Here's how the part is built. I have some questions about the finished solid (model axes, mm). A direction names the side the tool comes from. Round coordinates to 2 decimals unless told otherwise and drop trailing zeros. Write each loop counter-clockwise with the first axis right and the second up, starting at its lowest first coordinate (ties: lowest second). Pieces come first, ordered by that corner, then holes. Notation, with made-up numbers: (66.25, -6.75) - (81.25, -6.75) arc R24 cw to (81.25, 3.25) - close; hole circle Ø7 at (34, 40). An arc over 180 degrees is marked (long way). Write item = value, one per line. Start each with the question number.
Item 1: If I drill on line 1 along Y through (x, z) = (34.5, -9.25); line 2 along X through (y, z) = (-13, 1.25); line 3 along Z through (x, y) = (49, 34), over which ranges is the centre line in solid material (lowest first)? Write a range as [from, to].
Item 2: If we section it at C-C (z = -1.75): Please give me the cut outline in (x, y), and give its area (3 significant figures).
Item 3: If we section it at B-B (x = 4): Please give me the cut outline in (y, z), and give its area (3 significant figures).
Item 4: If we section it at D-D (y = -31): Please give me the cut outline in (x, z), and give its area (3 significant figures).
Item 5: Thinking about a two-plate mould opening in X: for faces 4 (the face through (33, 32.5, -13)), 5 (the face through (48, 20, -13)), 6 (the face through (18, -41, 1)), which applies, pulls with the +X half, pulls with the -X half, needs draft (parallel to the pull), parting line crosses it, or undercut?
Item 6: Which directions (+Z, -Z, +X, -X, +Y, -Y) give clear straight access to the entire face, cutting with the end or side of a thin tool? Please do faces 1 (the face through (0, -37.48, 2)), 2 (the face through (-18, -41, 1)), 3 (the face through (33, -34.5, -13)).
Item 7: If we section it at A-A (y = 11.5): Please give me the cut outline in (x, z), and give its area (3 significant figures).
Item 8: For P1, Ø5, axis at y = -22, z = -8.5, coming from the -X side; P2, Ø6, axis at x = 33.5, z = -15, coming from the -Y side; P3, Ø2, axis at y = -33.5, z = -13.5, coming from the +X side, each with a flat end and sliding along its axis, tell me the tip position at first contact or that it passes through.
```python
from build123d import *

# Parameters (mm, degrees)
EXTRUDE_1_DEPTH           = 3
SKETCH_3_W                = 12
SKETCH_3_H                = 2
SKETCH_3_W_2              = 2
SKETCH_3_H_2              = 6
SKETCH_3_H_3              = 10
EXTRUDE_2_DEPTH           = 26
CUT_EXTRUDE_5_DEPTH       = 80.722804771
CUT_EXTRUDE_5_DEPTH_BACK  = 3
SKETCH_5_W                = 4
SKETCH_5_H                = 4
SKETCH_5_W_2              = 16
CUT_EXTRUDE_6_DEPTH       = 3
SKETCH_6_W                = 70
SKETCH_6_H                = 50
CUT_EXTRUDE_7_DEPTH       = 10
CUT_EXTRUDE_10_DEPTH      = 80.722804771
CUT_EXTRUDE_10_DEPTH_BACK = 3


with BuildPart() as part:
    # 草图1 → 凸台-拉伸1 (new body)
    with BuildSketch(Plane.XY):
        with BuildLine():
            Line((-60, 34), (-60, -34))
            add(Edge.make_bspline(
                [(-60, -34), (0, -61.168399395), (60, -34)],
                knots=[0.841357477, 0.841357477, 0.841357477, 2.300235176, 2.300235176, 2.300235176], degree=2, weights=[1, 0.745548499, 1]))
            Line((60, -34), (60, 34))
            add(Edge.make_bspline(
                [(60, 34), (0, 61.168399395), (-60, 34)],
                knots=[3.982950131, 3.982950131, 3.982950131, 5.44182783, 5.44182783, 5.44182783], degree=2, weights=[1, 0.745548499, 1]))
        make_face()
    extrude(amount=EXTRUDE_1_DEPTH)

    # 草图3 → 凸台-拉伸2 (add)
    with BuildSketch(Plane(origin=(0, 0, 0), x_dir=(-1, 0, 0), z_dir=(0, 0, -1))):
        with Locations((-33, -33.5)):
            Rectangle(SKETCH_3_W, SKETCH_3_H)
        with Locations((47, -22.5)):
            Rectangle(SKETCH_3_W_2, SKETCH_3_H_2)
        with Locations((47, 22.5)):
            Rectangle(SKETCH_3_W_2, SKETCH_3_H_2)
        with Locations((-33, 33.5)):
            Rectangle(SKETCH_3_W, SKETCH_3_H)
        with Locations((-47, 20.5)):
            Rectangle(SKETCH_3_W_2, SKETCH_3_H_3)
    extrude(amount=EXTRUDE_2_DEPTH)

    # 草图4 → 切除-拉伸5 (cut, two sides: drawn at the far end of the back side and taken through both)
    with BuildSketch(Plane(origin=(0, 0, 0), x_dir=(-1, 0, 0), z_dir=(0, 0, -1)).offset(-CUT_EXTRUDE_5_DEPTH_BACK)):
        Polygon((-10, -284.821306472), (-10, -45.321810815), (-10, -37.47951977), (10, -37.47951977), (10, -45.321810815), (10, -284.821306472), (10, -763.820297787), (-10, -763.820297787), align=None)
    extrude(amount=CUT_EXTRUDE_5_DEPTH + CUT_EXTRUDE_5_DEPTH_BACK, mode=Mode.SUBTRACT)

    # 草图5 → 切除-拉伸6 (cut)
    with BuildSketch(Plane(origin=(0, 0, 0), x_dir=(-1, 0, 0), z_dir=(0, 0, -1))):
        with Locations((-16, -40.670164979)):
            Rectangle(SKETCH_5_W, SKETCH_5_H)
        with Locations((30, -36.670164979)):
            Rectangle(SKETCH_5_W_2, SKETCH_5_H)
        with Locations((16, -40.670164979)):
            Rectangle(SKETCH_5_W, SKETCH_5_H)
    extrude(amount=-CUT_EXTRUDE_6_DEPTH, mode=Mode.SUBTRACT)

    # 草图6 → 切除-拉伸7 (cut)
    with BuildSketch(Plane(origin=(0, 0, 0), x_dir=(-1, 0, 0), z_dir=(0, 0, -1))):
        with Locations((1, 1.9417e-05)):
            Rectangle(SKETCH_6_W, SKETCH_6_H)
    extrude(amount=-CUT_EXTRUDE_7_DEPTH, mode=Mode.SUBTRACT)

    # 草图7 → 切除-拉伸10 (cut, two sides: drawn at the far end of the back side and taken through both)
    with BuildSketch(Plane(origin=(0, 0, 0), x_dir=(-1, 0, 0), z_dir=(0, 0, -1)).offset(-CUT_EXTRUDE_10_DEPTH_BACK)):
        with BuildLine():
            Line((-47.914442952, 38.608895735), (-0.047490379, 38.608895735))
            Line((-0.047490379, 38.608895735), (47.914442952, 38.608895735))
            add(Edge.make_bspline(
                [(-47.914442952, 38.608895735), (0, 53.86648698), (47.914442952, 38.608895735)],
                knots=[4.161758339, 4.161758339, 4.161758339, 5.263019622, 5.263019622, 5.263019622], degree=2, weights=[0.945270908, 0.800277591, 0.945270908]))
        make_face()
    extrude(amount=CUT_EXTRUDE_10_DEPTH + CUT_EXTRUDE_10_DEPTH_BACK, mode=Mode.SUBTRACT)


solid = part.part
```
Reply:
q1.line_1 = [-34.5, -32.5], [32.5, 34.5]
q1.line_2 = [-60, -36], [34, 60]
q1.line_3 = [0, 3]
q2.outline = (-48, -25.5) - (-46, -25.5) - (-46, -19.5) - (-48, -19.5) - close; (-48, 19.5) - (-46, 19.5) - (-46, 25.5) - (-48, 25.5) - close; (27, -34.5) - (39, -34.5) - (39, -32.5) - (27, -32.5) - close; (27, 32.5) - (39, 32.5) - (39, 34.5) - (27, 34.5) - close; (46, 15.5) - (48, 15.5) - (48, 25.5) - (46, 25.5) - close
q2.area = 92.0 mm2
q3.outline = (-37.48, 0) - (-25, 0) - (-25, 3) - (-37.48, 3) - close; (25, 0) - (38.61, 0) - (38.61, 3) - (25, 3) - close
q3.area = 78.3 mm2
q4.outline = (-60, 0) - (60, 0) - (60, 3) - (-60, 3) - close
q4.area = 360 mm2
q5.face_4 = needs draft
q5.face_5 = pulls with the +X half
q5.face_6 = undercut
q6.face_1 = +Z, -Z, -Y
q6.face_2 = +Z, -Z
q6.face_3 = -Z, +X, -X, -Y
q7.outline = (-60, 0) - (-36, 0) - (-36, 3) - (-60, 3) - close; (34, 0) - (60, 0) - (60, 3) - (34, 3) - close
q7.area = 150 mm2
q8.P1 = -48
q8.P2 = -34.5
q8.P3 = 39
